Verification items for the finished model (mm, model axes). A direction names the side the tool comes from. Give positions to 0.01 mm unless a question says otherwise; leave off trailing zeros. Order: outer loops, then holes, each group sorted by start corner. A loop starts at its lowest first (then second) coordinate and runs counter-clockwise, first axis right, second up.
(1) Mould release check, pull along Z, two halves, no side actions. Record for faces 1 (the face through (19, 6.1, -29)), 2 (the face through (33, 1, -35)), 3 (the face through (64.487, 0.789, -32.195)), 4 (the face through (32, 7, -12.5)): pulls with the +Z half, pulls with the -Z half, needs draft (parallel to the pull), parting line crosses it, or undercut.
(2) Gauge pin test, flat ends, axial feed: pin 1 (3 mm diameter, centred on x = 34, y = 6, fed in from +Z); pin 2 (5 mm diameter, centred on x = 63, z = -32, fed in from +Y); pin 3 (2 mm diameter, centred on y = 4, z = -30, fed in from -X); pin 4 (4 mm diameter, centred on x = 43, z = -11.5, fed in from -Y). Record the tip position at first contact, or that the pin passes through.
(3) Sectioned sample at D-D on z = -14.5. Record the cut outline in (x, y), plus the area to 3 significant figures.
(4) Sectioned sample at B-B on z = -32. Record the cut outline in (x, y).
(5) Sectioned sample at A-A on x = 3. Record the cut outline in (y, z).
(6) Scan lines: L1, parallel to Z at x = 3, y = 0.8; L2, parallel to X at y = 1.05, z = -3; L3, parallel to X at y = 8.25, z = -17.5. Record each from-to range of solid material in increasing order.
(7) Access from +Z, -Z, +X, -X, +Y, -Y to the whole of each face (thin tool, end or side, straight path). Record for faces 5 (the face through (49, 5, -24)), 6 (the face through (24, 4, -29)), 7 (the face through (20, 5, -23)), 8 (the face through (33, 1, 0)), 9 (the face through (32, 7, -3)).
(8) Sectioned sample at C-C on y = 4. Record the cut outline in (x, z).
```python
from build123d import *

# Parameters (mm, degrees)
SKETCH1_W               = 66
SKETCH1_H               = 35
PCB_DEPTH               = 1.6
MOUNT_HOLE_1_DEPTH      = 75.723222629
MOUNT_HOLE_1_DEPTH_BACK = 75.723222629
SKETCH2_R               = 1.5
MOUNT_HOLE_2_DEPTH      = 75.723222629
MOUNT_HOLE_2_DEPTH_BACK = 75.723222629
SKETCH3_R               = 1.5
MOUNT_HOLE_3_DEPTH      = 75.723222629
MOUNT_HOLE_3_DEPTH_BACK = 75.723222629
SKETCH4_R               = 1.5
MOUNT_HOLE_4_DEPTH      = 75.723222629
MOUNT_HOLE_4_DEPTH_BACK = 75.723222629
SKETCH5_R               = 1.5
VOLTMETER_DISPLAY_START = 1.6
SKETCH6_W               = 23
SKETCH6_H               = 13
VOLTMETER_DISPLAY_DEPTH = 7
INDUCTOR_START          = 1.6
SKETCH7_W               = 12
SKETCH7_H               = 12
INDUCTOR_DEPTH          = 7
CAP_IN_START            = 1.6
SKETCH8_R               = 4
CAP_IN_DEPTH            = 12
CAP_OUT_START           = 1.6
SKETCH9_R               = 4
CAP_OUT_DEPTH           = 12
TRIM_POT_START          = 1.6
SKETCH10_W              = 9.5
SKETCH10_H              = 9.5
TRIM_POT_DEPTH          = 10
LM2596_START            = 1.6
SKETCH11_W              = 10
SKETCH11_H              = 8.5
LM2596_DEPTH            = 4.5


with BuildPart() as part:
    # Sketch1 → PCB (new body)
    with BuildSketch(Plane(origin=(0, 0, 0), x_dir=(1, 0, 0), z_dir=(0, 1, 0))):
        with Locations((33, 17.5)):
            Rectangle(SKETCH1_W, SKETCH1_H)
    extrude(amount=PCB_DEPTH)

    # Sketch2 → Mount_hole_1 (cut, two sides: drawn at the far end of the back side and taken through both)
    with BuildSketch(Plane(origin=(0, 0, 0), x_dir=(1, 0, 0), z_dir=(0, 1, 0)).offset(-MOUNT_HOLE_1_DEPTH_BACK)):
        with Locations(Location((3, 3, 0), (0, 0, 270))):
            Circle(SKETCH2_R)
    extrude(amount=MOUNT_HOLE_1_DEPTH + MOUNT_HOLE_1_DEPTH_BACK, mode=Mode.SUBTRACT)

    # Sketch3 → Mount_hole_2 (cut, two sides: drawn at the far end of the back side and taken through both)
    with BuildSketch(Plane(origin=(0, 0, 0), x_dir=(1, 0, 0), z_dir=(0, 1, 0)).offset(-MOUNT_HOLE_2_DEPTH_BACK)):
        with Locations(Location((63, 3, 0), (0, 0, 270))):
            Circle(SKETCH3_R)
    extrude(amount=MOUNT_HOLE_2_DEPTH + MOUNT_HOLE_2_DEPTH_BACK, mode=Mode.SUBTRACT)

    # Sketch4 → Mount_hole_3 (cut, two sides: drawn at the far end of the back side and taken through both)
    with BuildSketch(Plane(origin=(0, 0, 0), x_dir=(1, 0, 0), z_dir=(0, 1, 0)).offset(-MOUNT_HOLE_3_DEPTH_BACK)):
        with Locations(Location((3, 32, 0), (0, 0, 270))):
            Circle(SKETCH4_R)
    extrude(amount=MOUNT_HOLE_3_DEPTH + MOUNT_HOLE_3_DEPTH_BACK, mode=Mode.SUBTRACT)

    # Sketch5 → Mount_hole_4 (cut, two sides: drawn at the far end of the back side and taken through both)
    with BuildSketch(Plane(origin=(0, 0, 0), x_dir=(1, 0, 0), z_dir=(0, 1, 0)).offset(-MOUNT_HOLE_4_DEPTH_BACK)):
        with Locations(Location((63, 32, 0), (0, 0, 270))):
            Circle(SKETCH5_R)
    extrude(amount=MOUNT_HOLE_4_DEPTH + MOUNT_HOLE_4_DEPTH_BACK, mode=Mode.SUBTRACT)

    # Sketch6 → Voltmeter_display (add)
    with BuildSketch(Plane(origin=(0, 0, 0), x_dir=(1, 0, 0), z_dir=(0, 1, 0)).offset(VOLTMETER_DISPLAY_START)):
        with Locations((49.5, 17.5)):
            Rectangle(SKETCH6_W, SKETCH6_H)
    extrude(amount=VOLTMETER_DISPLAY_DEPTH)

    # Sketch7 → Inductor (add)
    with BuildSketch(Plane(origin=(0, 0, 0), x_dir=(1, 0, 0), z_dir=(0, 1, 0)).offset(INDUCTOR_START)):
        with Locations((20, 17)):
            Rectangle(SKETCH7_W, SKETCH7_H)
    extrude(amount=INDUCTOR_DEPTH)

    # Sketch8 → Cap_in (add)
    with BuildSketch(Plane(origin=(0, 0, 0), x_dir=(1, 0, 0), z_dir=(0, 1, 0)).offset(CAP_IN_START)):
        with Locations(Location((8, 22, 0), (0, 0, 90))):
            Circle(SKETCH8_R)
    extrude(amount=CAP_IN_DEPTH)

    # Sketch9 → Cap_out (add)
    with BuildSketch(Plane(origin=(0, 0, 0), x_dir=(1, 0, 0), z_dir=(0, 1, 0)).offset(CAP_OUT_START)):
        with Locations(Location((30, 27, 0), (0, 0, 90))):
            Circle(SKETCH9_R)
    extrude(amount=CAP_OUT_DEPTH)

    # Sketch10 → Trim_pot (add)
    with BuildSketch(Plane(origin=(0, 0, 0), x_dir=(1, 0, 0), z_dir=(0, 1, 0)).offset(TRIM_POT_START)):
        with Locations((31.75, 7.75)):
            Rectangle(SKETCH10_W, SKETCH10_H)
    extrude(amount=TRIM_POT_DEPTH)

    # Sketch11 → LM2596 (add)
    with BuildSketch(Plane(origin=(0, 0, 0), x_dir=(1, 0, 0), z_dir=(0, 1, 0)).offset(LM2596_START)):
        with Locations((19, 29.25)):
            Rectangle(SKETCH11_W, SKETCH11_H)
    extrude(amount=LM2596_DEPTH)


solid = part.part
```
Ans:
1. face 1: needs draft
1. face 2: pulls with the -Z half
1. face 3: undercut
1. face 4: undercut
2. pin 1: stops at z = -3
2. pin 2: stops at y = 1.6
2. pin 3: stops at x = 14
2. pin 4: stops at y = 0
3. outline: (0, 0) - (66, 0) - (66, 1.6) - (61, 1.6) - (61, 8.6) - (38, 8.6) - (38, 1.6) - (26, 1.6) - (26, 8.6) - (14, 8.6) - (14, 1.6) - (0, 1.6) - close
3. area: 351 mm2
4. outline: (0, 0) - (1.5, 0) - (1.5, 1.6) - (0, 1.6) - close; (4.5, 0) - (61.5, 0) - (61.5, 1.6) - (24, 1.6) - (24, 6.1) - (14, 6.1) - (14, 1.6) - (4.5, 1.6) - close; (64.5, 0) - (66, 0) - (66, 1.6) - (64.5, 1.6) - close
5. outline: (0, -35) - (1.6, -35) - (1.6, -33.5) - (0, -33.5) - close; (0, -30.5) - (1.6, -30.5) - (1.6, -4.5) - (0, -4.5) - close; (0, -1.5) - (1.6, -1.5) - (1.6, 0) - (0, 0) - close
6. L1: z = -35 to -33.5, -30.5 to -4.5, -1.5 to 0
6. L2: x = 0 to 1.5, 4.5 to 61.5, 64.5 to 66
6. L3: x = 14 to 26, 38 to 61
7. face 5: -Z, +X, +Y
7. face 6: -Z, +Y
7. face 7: +Y
7. face 8: +Z, +X, -X, +Y, -Y
7. face 9: +Z, +X, -X, +Y
8. outline: circle Ø8 at (8, -22); (14, -33.5) - (24, -33.5) - (24, -25) - (14, -25) - close; (14, -23) - (26, -23) - (26, -11) - (14, -11) - close; circle Ø8 at (30, -27); (27, -12.5) - (36.5, -12.5) - (36.5, -3) - (27, -3) - close; (38, -24) - (61, -24) - (61, -11) - (38, -11) - close
